Could you check a few things on this drawing? It's one solid part, dimensions in mm from its lowest x, y, z. A direction names the side the tool comes from. Round coordinates to 2 decimals unless told otherwise and drop trailing zeros. Write each loop counter-clockwise with the first axis right and the second up, starting at its lowest first coordinate (ties: lowest second). Pieces come first, ordered by that corner, then holes. Notation, with made-up numbers: (86.5, 85) -> (96.5, 85) arc R22 ccw to (96.5, 123) -> close; hole circle Ø11 at (8.5, -24.5). An arc over 180 degrees is marked (long way). Put each result on its own line as item: value. Start each with the question number.
1) I want a section at D-D, the plane x = 44. List the corners of the cut face in (y, z) for me, then the cut area to 3 significant figures.
2) I want a section at C-C, the plane y = 36. List the corners of the cut face in (x, z) for me.
3) We'd pull the mould along X, two halves only. Please class the marked faces 3, 4, 5 and 6: released by +X, released by -X, zero draft, split by the parting line, or undercut.
4) Will these pins go through, and if not, where does the flat tip stop? P1, Ø1.5, axis at x = 22, z = 0.5, coming from the -Y side; P2, Ø3, axis at y = 6.5, z = 3, coming from the -X side; P3, Ø1.5, axis at x = 23, z = 1.5, coming from the +Y side.
5) Which directions (+Z, -Z, +X, -X, +Y, -Y) give clear straight access to the entire face, cutting with the end or side of a thin tool? Please do the marked faces 1 and 2.
6) I want a section at A-A, the plane x = 25. List the corners of the cut face in (y, z) for me.
7) I want a section at B-B, the plane z = 2.4. List the corners of the cut face in (x, y) for me, then the cut area to 3 significant figures.
8) If I drill on line 1 along X through (y, z) = (5, 1.35); line 2 along Y through (x, z) = (25, 2.1); line 3 along Y through (x, z) = (6, 4.6), over which ranges is the centre line in solid material (lowest first)? Write a range as [from, to].
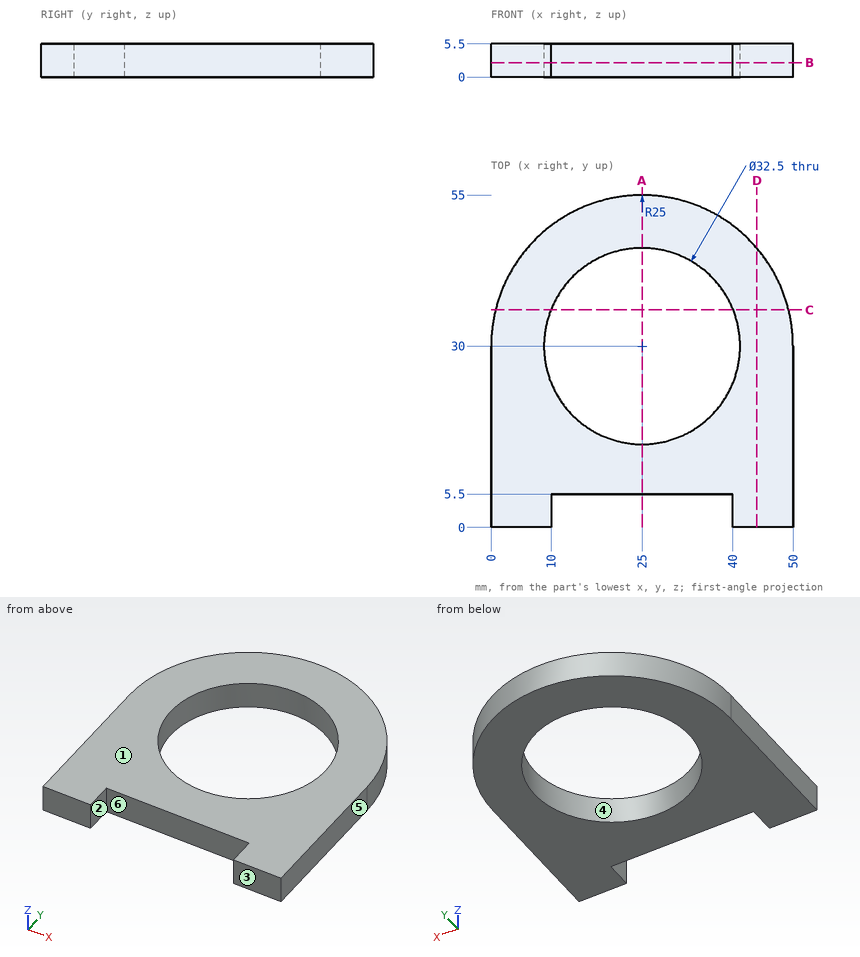
Findings:
1. outline: (0, 0) -> (46.25, 0) -> (46.25, 5.5) -> (0, 5.5) -> close
1. area: 254 mm2
2. outline: (0.73, 0) -> (9.9, 0) -> (9.9, 5.5) -> (0.73, 5.5) -> close; (40.1, 0) -> (49.27, 0) -> (49.27, 5.5) -> (40.1, 5.5) -> close
3. face 3: zero draft
3. face 4: undercut
3. face 5: released by +X
3. face 6: undercut
4. P1: stops at y = 5.5
4. P2: stops at x = 0
4. P3: stops at y = 54.97
5. face 1: +Z, +X, -X, +Y, -Y
5. face 2: +Z, -Z, -Y
6. outline: (5.5, 0) -> (13.75, 0) -> (13.75, 5.5) -> (5.5, 5.5) -> close; (46.25, 0) -> (55, 0) -> (55, 5.5) -> (46.25, 5.5) -> close
7. outline: (0, 0) -> (10, 0) -> (10, 5.5) -> (40, 5.5) -> (40, 0) -> (50, 0) -> (50, 30) arc R25 ccw to (0, 30) -> close; hole circle Ø32.5 at (25, 30)
7. area: 1,490 mm2
8. line 1: x = [0, 10], [40, 50]
8. line 2: y = [5.5, 13.75], [46.25, 55]
8. line 3: y = [0, 46.25]
